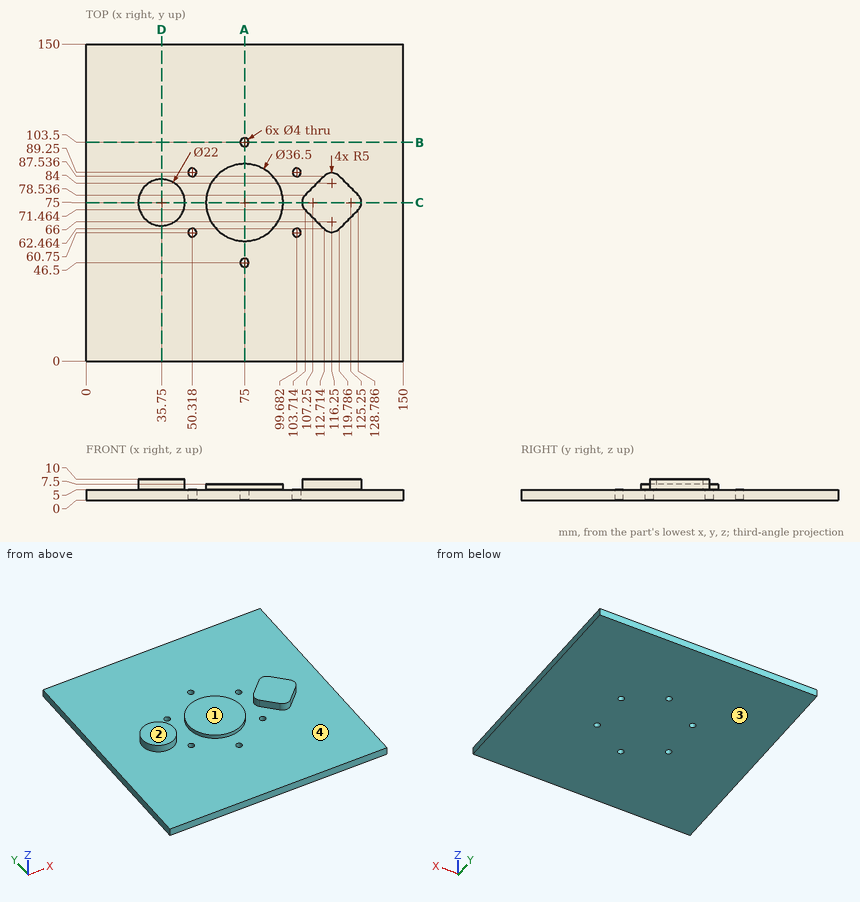
The figure shows three views and two pictorial views of one solid part (mm, origin at its lowest corner). Answer the questions. A direction names the side the tool comes from. Give positions to 0.01 mm unless a question says otherwise; leave off trailing zeros. Write each loop counter-clockwise with the first axis right and the second up, starting at its lowest first coordinate (ties: lowest second). Pieces come first, ordered by that corner, then holes. Notation, with made-up numbers: (63.25, 25) -> (80.25, 25) arc R21 cw to (80.25, 33) -> close; hole circle Ø6 at (13.5, 37.25). An arc over 180 degrees is marked (long way). Answer as a JSON object with one key per item and string values.
1) Section B-B on y = 103.5 is taken. Write down the section's boundary in (x, z), then the cut area to 3 significant figures.
Findings below:
{"outline": "(0, 0) -> (73, 0) -> (73, 5) -> (0, 5) -> close; (77, 0) -> (150, 0) -> (150, 5) -> (77, 5) -> close", "area": "730 mm^2"}
2) Straight lines are drawn through the part: probe 1 along Y at (x, z) = (75, 3.1); probe 2 along X at (y, z) = (77.5, 5.25); probe 3 along Z at (x, y) = (14.5, 86). For each, find the intervals that lie inside material, in ascending order. Write a range as from..to.
Findings below:
{"probe 1": "y = 0..44.5, 48.5..101.5, 105.5..150", "probe 2": "x = 25.04..46.46, 56.92..93.08, 102.92..129.58", "probe 3": "z = 0..5"}
3) Section A-A on x = 75 is taken. Write down the section's boundary in (y, z).
Findings below:
{"outline": "(0, 0) -> (44.5, 0) -> (44.5, 5) -> (0, 5) -> close; (48.5, 0) -> (101.5, 0) -> (101.5, 5) -> (93.25, 5) -> (93.25, 7.5) -> (56.75, 7.5) -> (56.75, 5) -> (48.5, 5) -> close; (105.5, 0) -> (150, 0) -> (150, 5) -> (105.5, 5) -> close"}
4) A tool of negligible diameter and unlimited length cuts with its end or side. For the marked faces 3 and 4, from which of +Z, -Z, +X, -X, +Y, -Y can it reach the whole face along a straight path? Write none if from no direction.
Findings below:
{"face 3": "-Z, +X, -X, +Y, -Y", "face 4": "+Z"}
5) For a pull along X with two mould halves and no side action, classify the marked faces 1 and 2 as pulls with the +X half, pulls with the -X half, needs draft (parallel to the pull), parting line crosses it, or undercut.
Findings below:
{"face 1": "undercut", "face 2": "needs draft"}
6) Flat-ended cylindrical pins translate along their axes: pin 1 Ø4 at (y, z) = (66.5, 8.5) entering from -X (1 decimal); pin 2 Ø5 at (x, y) = (99.68, 60.75) entering from +Z. Find the tip coordinate at first contact, or state that the pin passes through.
Findings below:
{"pin 1": "stops at x = 26.9", "pin 2": "stops at z = 5"}
7) Section D-D on x = 35.75 is taken. Write down the section's boundary in (y, z), then the cut area to 3 significant figures.
Findings below:
{"outline": "(0, 0) -> (150, 0) -> (150, 5) -> (86, 5) -> (86, 10) -> (64, 10) -> (64, 5) -> (0, 5) -> close", "area": "860 mm^2"}
8) Section C-C on y = 75 is taken. Write down the section's boundary in (x, z).
Findings below:
{"outline": "(0, 0) -> (150, 0) -> (150, 5) -> (130.25, 5) -> (130.25, 10) -> (102.25, 10) -> (102.25, 5) -> (93.25, 5) -> (93.25, 7.5) -> (56.75, 7.5) -> (56.75, 5) -> (46.75, 5) -> (46.75, 10) -> (24.75, 10) -> (24.75, 5) -> (0, 5) -> close"}
